```python
from build123d import *

# Parameters (mm, degrees)
SKETCH1_W                      = 7
SKETCH1_H                      = 4.8
BOSS_EXTRUDE1_DEPTH            = 70
CBORE_FOR_M2_SHCS1_D           = 2.4
CBORE_FOR_M2_SHCS1_CBORE_D     = 4.2
CBORE_FOR_M2_SHCS1_CBORE_DEPTH = 2.3


with BuildPart() as part:
    # Sketch1 → Boss-Extrude1 (new body)
    with BuildSketch(Plane.XY):
        with Locations((3.5, 2.4)):
            Rectangle(SKETCH1_W, SKETCH1_H)
    extrude(amount=BOSS_EXTRUDE1_DEPTH)

    # CBORE for M2 SHCS1 (through all)
    with Locations(Plane(origin=(0, 4.8, 0), x_dir=(1, 0, 0), z_dir=(0, 1, 0))):
        with Locations((3.5, -65), (3.5, -50), (3.5, -35), (3.5, -20), (3.5, -5)):
            CounterBoreHole(CBORE_FOR_M2_SHCS1_D / 2, CBORE_FOR_M2_SHCS1_CBORE_D / 2, CBORE_FOR_M2_SHCS1_CBORE_DEPTH)


solid = part.part
```
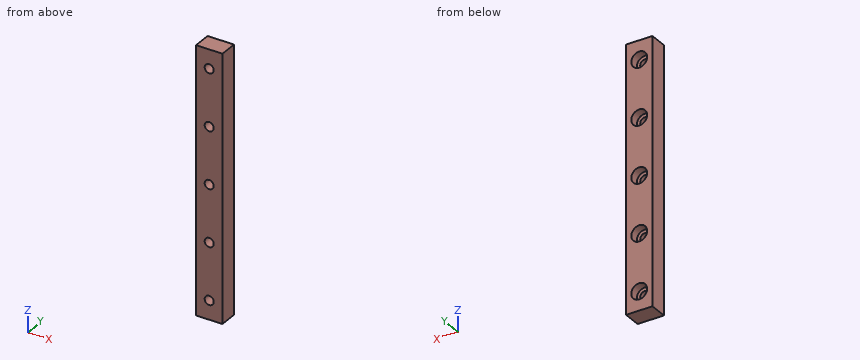
Can you work these out from the model? Positions are in its coordinate system, mm. Round coordinates to 2 decimals unless told otherwise and drop trailing zeros. Order: outer loops, then holes, each group sorted by start corner. A loop starts at its lowest first (then second) coordinate and runs counter-clockwise, first axis right, second up.
(1) If I drill on L1, parallel to Z at x = 3.5, y = 0.8; L2, parallel to X at y = 3.5, z = 65; L3, parallel to X at y = 1.55, z = 50, over which ranges is the centre line in solid material (lowest first)?
Results are:
L1: z = 0 to 3.8, 6.2 to 18.8, 21.2 to 33.8, 36.2 to 48.8, 51.2 to 63.8, 66.2 to 70
L2: x = 0 to 1.4, 5.6 to 7
L3: x = 0 to 2.3, 4.7 to 7
(2) If we section it at A-A (z = 35): Please give me the cut outline in (x, y).
Results are:
outline: (0, 0) - (2.3, 0) - (2.3, 2.5) - (1.4, 2.5) - (1.4, 4.8) - (0, 4.8) - close; (4.7, 0) - (7, 0) - (7, 4.8) - (5.6, 4.8) - (5.6, 2.5) - (4.7, 2.5) - close
(3) I'm going to push flat-ended pins straight in: pin 1 (1.4 mm diameter, centred on x = 3.5, z = 50, fed in from +Y); pin 2 (2.5 mm diameter, centred on x = 3.5, z = 20, fed in from +Y). Where does each tip first touch, or does it pass through?
Results are:
pin 1: passes through
pin 2: stops at y = 2.5
(4) If we section it at B-B (x = 3.5): Count the separate pieces of the cut face and the enclosed holes in it, plus the area to 3 significant figures.
Results are:
separate pieces: 6
enclosed holes: 0
area: 258 mm2
